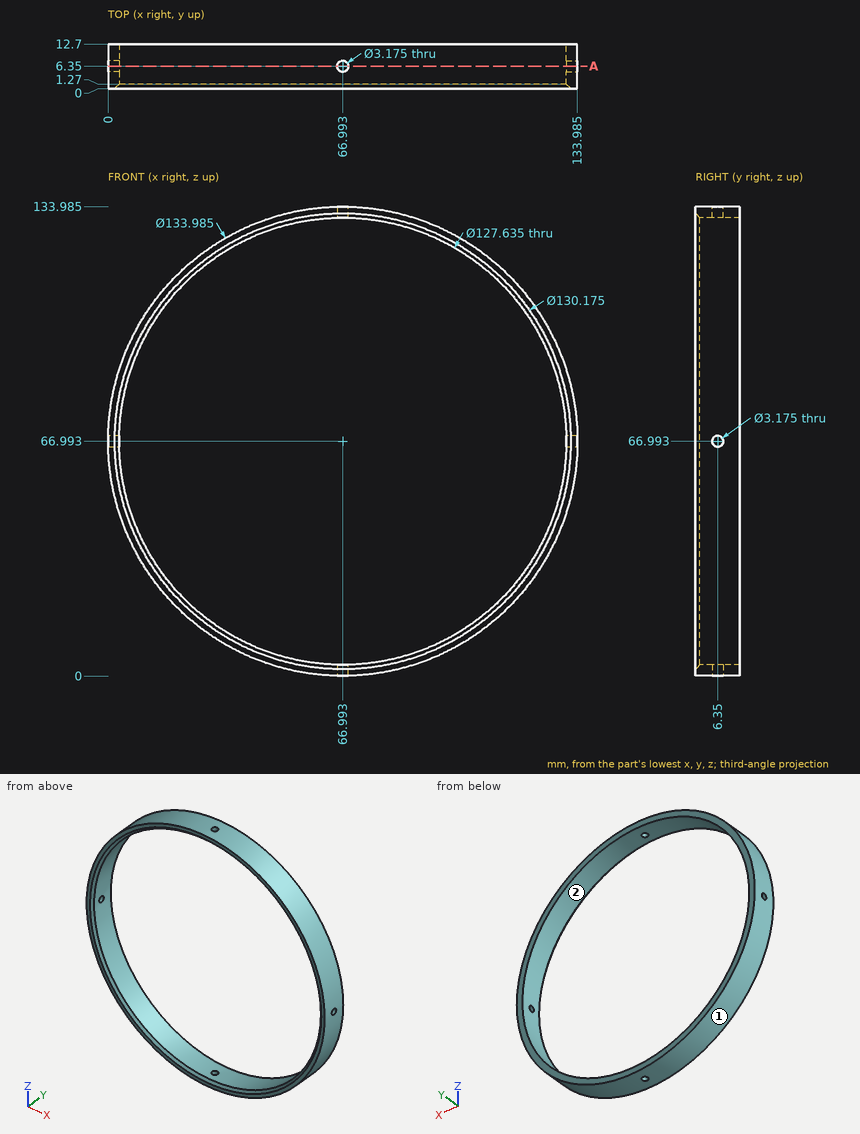
Print and shaded views of the part. All mm, measured from the part's lowest x, y and z. Round coordinates to 2 decimals unless told otherwise and drop trailing zeros. Write each loop counter-clockwise with the first axis right and the second up, starting at its lowest first coordinate (ties: lowest second). Pieces come first, ordered by that corner, then holes.
Item 1: Cut at A-A, the plane y = 6.35. Give the cut face in (x, z) (1 decimal).
Results:
outline: (0, 65.4) arc R67 ccw to (65.4, 0) - (65.4, 3.2) arc R63.8 cw to (3.2, 65.4) - close; (0, 68.6) - (3.2, 68.6) arc R63.8 cw to (65.4, 130.8) - (65.4, 134) arc R67 ccw to start; (68.6, 0) arc R67 ccw to (134, 65.4) - (130.8, 65.4) arc R63.8 cw to (68.6, 3.2) - close; (68.6, 130.8) arc R63.8 cw to (130.8, 68.6) - (134, 68.6) arc R67 ccw to (68.6, 134) - close
Item 2: Drop flat-ended pins along their axis: pin 1 Ø5 at (x, y) = (97, 9) entering from -Z; pin 2 Ø3.5 at (y, z) = (6.35, 66.99) entering from +X (1 decimal); pin 3 Ø2 at (x, y) = (28, 10.5) entering from +Z; pin 4 Ø5 at (y, z) = (4.5, 18.5) entering from +X. Give the stop position or say it passes through.
Results:
pin 1: stops at z = 5.91
pin 2: stops at x = 134
pin 3: stops at z = 122.17
pin 4: stops at x = 115.7
Item 3: Probe L1, parallel to X at y = 4, z = 68; L2, parallel to Z at x = 49.5, y = 3 (1 decimal); L3, parallel to X at y = 2, z = 29 (1 decimal). List the from-to ranges inside material, lowest first.
Results:
L1: x = 0.01 to 3.18, 130.8 to 133.98
L2: z = 2.3 to 5.6, 128.4 to 131.7
L3: x = 11.8 to 15.7, 118.3 to 122.2
Item 4: Two-plate mould, pull along Z, no slides. Class the marked faces 1 and 2: +Z half, -Z half, draft (parallel to the pull), parting line (faces both ways), or undercut.
Results:
face 1: parting line
face 2: undercut
